The listing builds one solid part. Answer for the finished solid, in the listing's coordinates (mm). A direction names the side the tool comes from. Round coordinates to 2 decimals unless told otherwise and drop trailing zeros. Write each loop counter-clockwise with the first axis right and the second up, starting at its lowest first coordinate (ties: lowest second). Pieces come first, ordered by that corner, then holes.
(1) The mould has two halves that part along X. Classify faces 1 (the face through (-13.887, -10.648, 1.479)), 2 (the face through (-0.37, 5.84, 10.14)), 3 (the face through (11, 8, 17)), 4 (the face through (-5.71, -5.26, 10.14)): +X half, -X half, draft (parallel to the pull), parting line (faces both ways), or undercut.
(2) A cutting plane is placed at B-B, the plane x = 0. Give the vertices of the cut face in (y, z), and give its area (3 significant figures).
(3) Each of these flat-tipped pins is pushed along its axis until it touches: pin 1 Ø5 at (y, z) = (-8.5, 18) entering from +X; pin 2 Ø2 at (x, y) = (0, 7.5) entering from +Z; pin 3 Ø1 at (y, z) = (-9, 8) entering from -X; pin 4 Ø1.5 at (x, z) = (-6.5, 7) entering from -Y. Where does it stop, or does it pass through?
(4) A cutting plane is placed at A-A, the plane y = 0. Give the vertices of the cut face in (x, z), and give its area (3 significant figures).
(5) A cutting plane is placed at C-C, the plane z = 1.5. Give the vertices of the cut face in (x, y), and give its area (3 significant figures).
(6) For faces 5 (the face through (11, 8, 3)), 6 (the face through (0, -4, 0)), determine the directions among +Z, -Z, +X, -X, +Y, -Y from which every point of the face is accessible in a straight line to the end or side of a thin tool.
(7) Find the intervals of material crossed by probe 1 along Y at (x, z) = (0, 5.5); probe 2 along Z at (x, y) = (12.5, 9); probe 3 along Y at (x, z) = (6.5, 9.75), in increasing order.
(8) A cutting plane is placed at D-D, the plane x = -6.5. Give the vertices of the cut face in (y, z), and give its area (3 significant figures).
from build123d import *

# Parameters (mm, degrees)
ESQUISSE1_R             = 17.5
BOSS_EXTRU_1_DEPTH      = 20
ESQUISSE3_W             = 14
ESQUISSE3_H             = 5
ESQUISSE4_R             = 2.5
ENL_V_MAT_EXTRU_1_DEPTH = 20
D_GAGEMENT_M31_D        = 3.4


with BuildPart() as part:
    # Esquisse1 → Boss.-Extru.1 (new body)
    with BuildSketch(Plane.XY):
        Circle(ESQUISSE1_R)
    extrude(amount=BOSS_EXTRU_1_DEPTH)

    # Esquisse3 → Enlèvement de matière-Révolution2 (revolve, cut)
    with BuildSketch(Plane(origin=(0, 0, 0), x_dir=(0, 0, -1), z_dir=(1, 0, 0)), mode=Mode.PRIVATE) as enl_vement_de_mati_re_r_volution2_sk:
        with Locations((-10, 15)):
            Rectangle(ESQUISSE3_W, ESQUISSE3_H)
    revolve(enl_vement_de_mati_re_r_volution2_sk.sketch.rotate(Axis((0, 0, 0), (0, 0, 1)), 90), axis=Axis((0, 0, 0), (0, 0, 1)), mode=Mode.SUBTRACT)

    # Esquisse4 → Enlèv. mat.-Extru.1 (cut)
    with BuildSketch(Plane(origin=(0, 0, 0), x_dir=(-1, 0, 0), z_dir=(0, 0, -1))):
        Circle(ESQUISSE4_R)
    extrude(amount=-ENL_V_MAT_EXTRU_1_DEPTH, mode=Mode.SUBTRACT)

    # Dégagement M31 (through all)
    with Locations(Plane(origin=(0, 0, 0), x_dir=(-1, 0, 0), z_dir=(0, 0, -1))):
        with Locations((0, 7.5), (6.495190528, -3.75), (-6.495190528, -3.75), (0, 0)):
            Hole(D_GAGEMENT_M31_D / 2)


solid = part.part
Solutions:
1. face 1: parting line
1. face 2: undercut
1. face 3: draft
1. face 4: undercut
2. outline: (-17.5, 0) - (-2.5, 0) - (-2.5, 20) - (-17.5, 20) - (-17.5, 17) - (-12.5, 17) - (-12.5, 3) - (-17.5, 3) - close; (2.5, 0) - (5.8, 0) - (5.8, 20) - (2.5, 20) - close; (9.2, 0) - (17.5, 0) - (17.5, 3) - (12.5, 3) - (12.5, 17) - (17.5, 17) - (17.5, 20) - (9.2, 20) - close
2. area: 392 mm2
3. pin 1: stops at x = 16.44
3. pin 2: passes through
3. pin 3: stops at x = -9.17
3. pin 4: stops at y = -11.1
4. outline: (-17.5, 0) - (-2.5, 0) - (-2.5, 20) - (-17.5, 20) - (-17.5, 17) - (-12.5, 17) - (-12.5, 3) - (-17.5, 3) - close; (2.5, 0) - (17.5, 0) - (17.5, 3) - (12.5, 3) - (12.5, 17) - (17.5, 17) - (17.5, 20) - (2.5, 20) - close
4. area: 460 mm2
5. outline: circle Ø35 at (0, 0); hole circle Ø3.4 at (-6.5, -3.75); hole circle Ø5 at (0, 0); hole circle Ø3.4 at (0, 7.5); hole circle Ø3.4 at (6.5, -3.75)
5. area: 915 mm2
6. face 5: none
6. face 6: -Z, +X, -X, +Y, -Y
7. probe 1: y = -12.5 to -2.5, 2.5 to 5.8, 9.2 to 12.5
7. probe 2: z = 0 to 3, 17 to 20
7. probe 3: y = -10.68 to -5.45, -2.05 to 10.68
8. outline: (-16.25, 0) - (-5.45, 0) - (-5.45, 20) - (-16.25, 20) - (-16.25, 17) - (-10.68, 17) - (-10.68, 3) - (-16.25, 3) - close; (-2.05, 0) - (16.25, 0) - (16.25, 3) - (10.68, 3) - (10.68, 17) - (16.25, 17) - (16.25, 20) - (-2.05, 20) - close
8. area: 426 mm2
